```python
from build123d import *

# Parameters (mm, degrees)
F0_W     = 127
F0_H     = 134.62
F1_DEPTH = 152.4
F2_T     = -10.16
F4_DEPTH = 127


with BuildPart() as f1:
    # F0 (on Front) → F1 (new body)
    with BuildSketch(Plane.XZ):
        with Locations((63.5, 67.31)):
            Rectangle(F0_W, F0_H)
    extrude(amount=F1_DEPTH)

    # F2
    f2_openings = [f1.faces().sort_by_distance(p)[0] for p in [
        (63.5, -152.4, 67.31),
    ]]
    offset(amount=F2_T, openings=f2_openings)

    # F3 (on Right) → F4 (join, through all)
    with BuildSketch(Plane.YZ):
        Polygon((-152.4, -87.988181), (0, 0), (-152.4, 0), align=None)
    extrude(amount=F4_DEPTH)


solid = f1.part
```
The model under review builds one solid part; all positions refer to its coordinate system, in mm. A direction names the side the tool comes from. Round coordinates to 2 decimals unless told otherwise and drop trailing zeros. Loops run counter-clockwise (first coordinate to the right, second up) from the corner with the lowest first, then second, coordinate; pieces in that order, holes last. Notation, with made-up numbers: M -21.5,-14.5 L -15.5,-14.5 A15 cw -15.5,-2.5 Z; hole C 59.5,11 d4. An arc over 180 degrees is marked long. Write item = value, one per line.
Item 1: Take a section at B-B on y = -60.5. Write out the cut boundary in (x, z).
Return value:
outline = M 0,-34.93 L 127,-34.93 L 127,134.62 L 0,134.62 Z; hole M 10.16,10.16 L 116.84,10.16 L 116.84,124.46 L 10.16,124.46 Z
Item 2: Insertion check: P1, Ø6, axis at x = 43.5, y = -63, coming from the -Z side; P2, Ø8, axis at x = 29, y = -66.5, coming from the -Z side. Each pin has a flat end and moves straight along its axis. Give the tip position at first contact, or say it passes through.
Return value:
P1 = -38.11
P2 = -40.7
Item 3: Take a section at C-C on z = 37.5. Write out the cut boundary in (x, y).
Return value:
outline = M 0,-152.4 L 10.16,-152.4 L 10.16,-10.16 L 116.84,-10.16 L 116.84,-152.4 L 127,-152.4 L 127,0 L 0,0 Z
Item 4: For line 1 (X direction, y = -82.5, z = 36.5); line 2 (Y direction, x = 44, z = 43); line 3 (Z direction, x = 77, y = -55), list the stretches that pass through material, from the lowest coordinate up. Write a range as [from, to].
Return value:
line_1 = [0, 10.16], [116.84, 127]
line_2 = [-10.16, 0]
line_3 = [-31.75, 10.16], [124.46, 134.62]
Item 5: The part is to be moulded in two halves that separate along Z. For faces 1 (the flat face through (62.61, -77.27, -44.61)), 2 (the flat face through (63, -152.4, -25)), 3 (the flat face through (116.84, -80, 67)), say which applies: released by +Z, released by -Z, zero draft, split by the parting line, or undercut.
Return value:
face_1 = released by -Z
face_2 = zero draft
face_3 = undercut
Item 6: Take a section at A-A on x = 54.5. Write out the cut boundary in (y, z), then the cut area to 3 significant figures.
Return value:
outline = M -152.4,-87.99 L 0,0 L 0,134.62 L -152.4,134.62 L -152.4,124.46 L -10.16,124.46 L -10.16,10.16 L -152.4,10.16 Z
area = 11,000 mm2
Item 7: Take a section at D-D on y = -136. Write out the cut boundary in (x, z), then the cut area to 3 significant figures.
Return value:
outline = M 0,-78.52 L 127,-78.52 L 127,134.62 L 0,134.62 Z; hole M 10.16,10.16 L 116.84,10.16 L 116.84,124.46 L 10.16,124.46 Z
area = 14,900 mm2
Item 8: Machinability: for faces 4 (the flat face through (63, -75, 134.62)), 5 (the flat face through (63, -10.16, 68)), which of the approach directions +Z, -Z, +X, -X, +Y, -Y give a long, thin tool a straight path to every point of the face, cutting with its end or side? Answer none if there is none.
Return value:
face_4 = +Z, +X, -X, +Y, -Y
face_5 = -Y
